Can you work these out from the model? Positions are in its coordinate system, mm. A direction names the side the tool comes from. Give positions to 0.01 mm unless a question says otherwise; leave off trailing zeros. Loops run counter-clockwise (first coordinate to the right, second up) from the corner with the lowest first, then second, coordinate; pieces in that order, holes last. Notation, with made-up numbers: (26.25, -37) - (45.25, -37) arc R24 ccw to (45.25, -5) - close; hole circle Ø1 at (0, -27.75). An arc over 180 degrees is marked (long way). Answer as a JSON object with one key per item and string values.
```python
from build123d import *

# Parameters (mm, degrees)
SKETCH2_W     = 0.6
SKETCH2_H     = 4.118227863
SKETCH2_H_2   = 1.3
SKETCH10_R    = 0.6
CHAMFER1_SIZE = 0.15


with BuildPart() as part:
    # Sketch1 → Revolve1 (revolve)
    with BuildSketch(Plane.XY, mode=Mode.PRIVATE) as revolve1_sk:
        with BuildLine():
            Line((1.626095531, 4.986801801), (10.92153598, 4.986801801))
            Line((10.92153598, 4.986801801), (10.92153598, 5.588836435))
            add(Edge.make_bspline(
                [(10.00241881, 6.452631049), (10.113570909, 5.637430805), (10.92153598, 5.588836435)],
                knots=[0, 0, 0, 1, 1, 1], degree=2))
            Line((10.00241881, 6.452631049), (9.732019166, 6.452631049))
            Line((9.732019166, 6.452631049), (9.732019166, 5.958857786))
            ThreePointArc((9.732019166, 5.958857786), (9.688976654, 5.854943969), (9.585062838, 5.811901457))
            Line((9.585062838, 5.811901457), (8.673933602, 5.811901457))
            ThreePointArc((8.673933602, 5.811901457), (8.56170668, 5.85838737), (8.515220767, 5.970614292))
            Line((8.515220767, 5.970614292), (8.515220767, 6.452631049))
            Line((8.515220767, 6.452631049), (8.072127944, 6.452631049))
            Line((8.072127944, 6.452631049), (8.072127944, 6.272997822))
            Line((8.072127944, 6.272997822), (2.861199395, 6.272997822))
            add(Edge.make_bspline(
                [(1.626095531, 4.986801801), (1.568844138, 5.647468558), (2.210932821, 6.320979116), (2.861199395, 6.272997822)],
                knots=[0, 0, 0, 0, 1, 1, 1, 1], degree=3))
        make_face()
    revolve(revolve1_sk.sketch.rotate(Axis((1.626095531, 4.986801801, 0), (1, 0, 0)), 90), axis=Axis((1.626095531, 4.986801801, 0), (1, 0, 0)))



with BuildPart() as body_2:
    # Sketch2 → Revolve2 (revolve)
    with BuildSketch(Plane.XY, mode=Mode.PRIVATE) as revolve2_sk:
        with Locations((12.178892064, 2.059113932)):
            Rectangle(SKETCH2_W, SKETCH2_H)
        with Locations((12.178892064, -0.65)):
            Rectangle(SKETCH2_W, SKETCH2_H_2)
    revolve(revolve2_sk.sketch.rotate(Axis((11.878892064, 4.118227863, 0), (0, -1, 0)), 90), axis=Axis((11.878892064, 4.118227863, 0), (0, -1, 0)))


with BuildPart() as part_1:
    add(part.part)

    add(body_2.part)  # Sweep1 merges body 2
    # Sweep1: sweep along a path in Sketch3
    with BuildLine() as sweep1_path:  # in the path sketch's own coordinates; laid on its plane below (add() does not lay a ready-made edge on the line's plane)
        add(Edge.make_bspline(
            [(10.92153598, 4.986801801), (11.822294838, 5.066317243), (11.878892064, 4.118227863)],
            knots=[0, 0, 0, 1, 1, 1], degree=2))
    # Sketch10 → Sweep1 (sweep)
    with BuildSketch(Plane(origin=(0, 4.118227863, 0), x_dir=(1, 0, 0), z_dir=(0, 1, 0))):
        with Locations((11.878892064, 0)):
            Circle(SKETCH10_R)
    sweep(path=Plane.XY * sweep1_path.line)

    # Chamfer1
    chamfer1_edges = [part_1.edges().sort_by_distance(p)[0] for p in [
        (11.878892064, -1.3, -0.6),
    ]]
    chamfer(chamfer1_edges, length=CHAMFER1_SIZE)


solid = part_1.part
```
1) I'm going to push a flat-ended pin straight in: P1, Ø0.6, axis at y = 5, z = 0, coming from the +X side. Where does the tip first touch, or does it pass through?
Check sheet entries:
{"P1": "x = 12.37"}
2) Imagine slicing it at A-A on x = 3. Write out the boundary of the cut face in (y, z), and give its area (3 significant figures).
Check sheet entries:
{"outline": "circle Ø2.57 at (4.99, 0)", "area": "5.20 mm2"}
3) Which directions (+Z, -Z, +X, -X, +Y, -Y) give clear straight access to the entire face, cutting with the end or side of a thin tool? Please do faces 1 (the cylindrical face through (11.284, 1.521, -0.078)), 2 (the cylindrical face through (9.12, 5.79, -0.18)).
Check sheet entries:
{"face 1": "-Y", "face 2": "none"}
4) Imagine slicing it at B-B on x = 8.25. Write out the boundary of the cut face in (y, z), and give its area (3 significant figures).
Check sheet entries:
{"outline": "circle Ø2.93 at (4.99, 0)", "area": "6.75 mm2"}
5) I need wall thicknesses on L1, parallel to X at y = 1, z = 0; L2, parallel to Z at x = 9, y = 5 (3 decimals); L3, parallel to X at y = 2.5, z = 0.4. Which ranges of each line are inside material? Lowest first, please.
Check sheet entries:
{"L1": "11.28 to 12.48", "L2": "-0.825 to 0.825", "L3": "11.43 to 12.33"}
